Can you work these out from the drawing? Everything is in mm from the part's minimum corner. A direction names the side the tool comes from. Round coordinates to 2 decimals unless told otherwise and drop trailing zeros. Loops run counter-clockwise (first coordinate to the right, second up) from the corner with the lowest first, then second, coordinate; pieces in that order, holes last. Notation, with made-up numbers: M -31.75,40.5 L -2.75,40.5 A32 ccw -2.75,76.5 Z; hole C -21,69 d3. An arc over 180 degrees is marked long. Use a Markdown table: item, result.
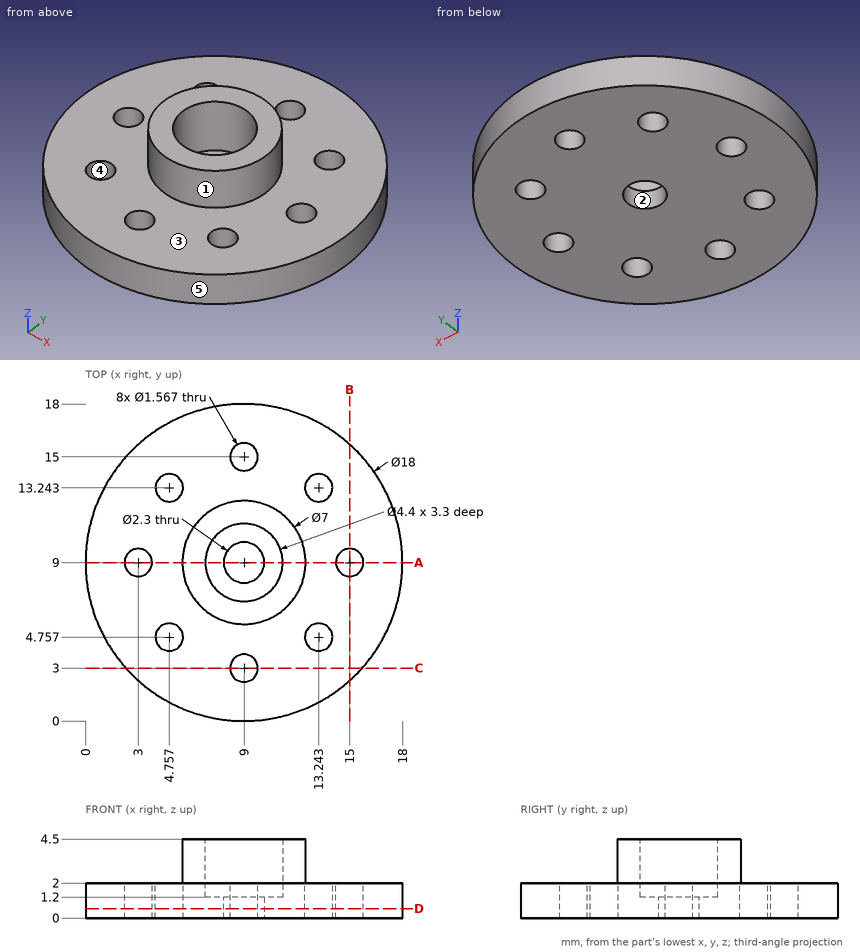
Q1. Imagine slicing it at D-D, the plane z = 0.55. Give the number of separate pieces and of enclosed holes in the cut face, then the cut area to 3 significant figures.
Return value:
| item | result |
|---|---|
| separate pieces | 1 |
| enclosed holes | 9 |
| area | 235 mm^2 |
Q2. I need wall thicknesses on line 1 (Y direction, x = 9, z = 0.85); line 2 (Y direction, x = 9.25, z = 1.7) (1 decimal); line 3 (Y direction, x = 9, z = 3.4). Which ranges of each line are inside material? Lowest first, please. Write a range as from..to.
Return value:
| item | result |
|---|---|
| line 1 | y = 0..2.22, 3.78..7.85, 10.15..14.22, 15.78..18 |
| line 2 | y = 0..2.3, 3.7..6.8, 11.2..14.3, 15.7..18 |
| line 3 | y = 5.5..6.8, 11.2..12.5 |
Q3. Imagine slicing it at A-A, the plane y = 9. Please give me the cut outline in (x, z).
Return value:
| item | result |
|---|---|
| outline | M 0,0 L 2.22,0 L 2.22,2 L 0,2 Z; M 3.78,0 L 7.85,0 L 7.85,1.2 L 6.8,1.2 L 6.8,4.5 L 5.5,4.5 L 5.5,2 L 3.78,2 Z; M 10.15,0 L 14.22,0 L 14.22,2 L 12.5,2 L 12.5,4.5 L 11.2,4.5 L 11.2,1.2 L 10.15,1.2 Z; M 15.78,0 L 18,0 L 18,2 L 15.78,2 Z |
Q4. Will these pins go through, and if not, where does the flat tip stop? P1, Ø1.4, axis at x = 3, y = 9, coming from the +Z side; P2, Ø1, axis at x = 3.5, y = 3, coming from the +Z side; P3, Ø1.5, axis at y = 5.5, z = 0.5, coming from the +X side.
Return value:
| item | result |
|---|---|
| P1 | passes through |
| P2 | stops at z = 2 |
| P3 | stops at x = 17.57 |
Q5. For the marked faces 1 and 2, which set-ups out of +Z, -Z, +X, -X, +Y, -Y let a thin tool reach every point of the face, with its end or its side?
Return value:
| item | result |
|---|---|
| face 1 | +Z |
| face 2 | +Z, -Z |
Q6. Imagine slicing it at B-B, the plane x = 15. Please give me the cut outline in (y, z), then the cut area to 3 significant figures.
Return value:
| item | result |
|---|---|
| outline | M 2.29,0 L 8.22,0 L 8.22,2 L 2.29,2 Z; M 9.78,0 L 15.71,0 L 15.71,2 L 9.78,2 Z |
| area | 23.7 mm^2 |
Q7. We'd pull the mould along Y, two halves only. Please class the marked faces 3, 4 and 5: pulls with the +Y half, pulls with the -Y half, needs draft (parallel to the pull), parting line crosses it, or undercut.
Return value:
| item | result |
|---|---|
| face 3 | needs draft |
| face 4 | undercut |
| face 5 | parting line crosses it |
